The listing builds one solid part. Answer for the finished solid, in the listing's coordinates (mm). A direction names the side the tool comes from. Round coordinates to 2 decimals unless told otherwise and drop trailing zeros. Write each loop counter-clockwise with the first axis right and the second up, starting at its lowest first coordinate (ties: lowest second). Pieces come first, ordered by that corner, then holes.
from build123d import *

# Parameters (mm, degrees)
F0_W     = 75.017012
F0_H     = 75.16501
F1_DEPTH = 13.462
F2_R     = 13.296545
F3_DEPTH = 18.542
F5_DEPTH = 21.336


with BuildPart() as f1:
    # F0 (on Top) → F1 (new body)
    with BuildSketch(Plane.XY):
        Rectangle(F0_W, F0_H)
    extrude(amount=F1_DEPTH)

    # F2 (on face) → F3 (join)
    with BuildSketch(Plane.XY.offset(13.462)):
        Circle(F2_R)
    extrude(amount=F3_DEPTH)

    # F4 (on Front) → F5 (cut, symmetric)
    with BuildSketch(Plane.XZ):
        Polygon((14.776042, 34.1333), (-13.614605, 32.584719), (14.776042, 17.098911), align=None)
    extrude(amount=F5_DEPTH, both=True, mode=Mode.SUBTRACT)


solid = f1.part
1. Section C-C on z = 20.5 is taken. Determine the outline of the cut face in (x, y).
Geometry says:
outline: (8.54, -10.19) - (8.54, 10.19) arc R13.3 ccw (long way) to start
2. Straight lines are drawn through the part: line 1 along Z through (x, y) = (-28, 14); line 2 along X through (y, z) = (-6, 23); line 3 along X through (y, z) = (1, 30.5). For each, find the intervals that lie inside material, in ascending order.
Geometry says:
line 1: z = 0 to 13.46
line 2: x = -11.87 to 3.96
line 3: x = -13.26 to -9.79
3. Section B-B on x = -9 is taken. Determine the outline of the cut face in (y, z).
Geometry says:
outline: (-37.58, 0) - (37.58, 0) - (37.58, 13.46) - (9.79, 13.46) - (9.79, 30.07) - (-9.79, 30.07) - (-9.79, 13.46) - (-37.58, 13.46) - close
4. Given pin 1 (4 mm diameter, centred on x = -29, y = 26, fed in from +Z); pin 2 (12 mm diameter, centred on x = 2, z = 28.5, fed in from -Y), each flat-ended and moving along its own axis, determine where each tip first touches the part or whether it passes through.
Geometry says:
pin 1: stops at z = 13.46
pin 2: stops at y = -13.3
5. A tool of negligible diameter and unlimited length cuts with its end or side. For faces 1 (the face through (-1, 37.583, 7)), 2 (the face through (-13.284, 0.585, 20.543)), from which of +Z, -Z, +X, -X, +Y, -Y can it reach the whole face along a straight path? Write none if from no direction.
Geometry says:
face 1: +Z, -Z, +X, -X, +Y
face 2: +Z
6. Section A-A on y = 0 is taken. Determine the outline of the cut face in (x, z), plus the area to 3 significant figures.
Geometry says:
outline: (-37.51, 0) - (37.51, 0) - (37.51, 13.46) - (13.3, 13.46) - (13.3, 17.91) - (-12.55, 32) - (-13.3, 32) - (-13.3, 13.46) - (-37.51, 13.46) - close
area: 1,320 mm2
7. Section D-D on x = 0 is taken. Determine the outline of the cut face in (y, z).
Geometry says:
outline: (-37.58, 0) - (37.58, 0) - (37.58, 13.46) - (13.3, 13.46) - (13.3, 25.16) - (-13.3, 25.16) - (-13.3, 13.46) - (-37.58, 13.46) - close
